```python
from build123d import *

# Parameters (mm, degrees)
EXTRUDE_1_DEPTH = 75
FILLET_1_R      = 3


with BuildPart() as part:
    # Эскиз1 → Вытянуть-Тонкостенный1 (new, symmetric)
    with BuildSketch(Plane.XY):
        Polygon((0, 0), (20, 0), (20, 53), (0, 53), (0, 50), (17, 50), (17, 3), (0, 3), align=None)
    extrude(amount=EXTRUDE_1_DEPTH, both=True)

    # Скругление1
    fillet_1_edges = [part.edges().sort_by_distance(p)[0] for p in [
        (17, 3, 0),
        (17, 50, 0),
    ]]
    fillet(fillet_1_edges, radius=FILLET_1_R)


solid = part.part
```
The model under review builds one solid part; all positions refer to its coordinate system, in mm. A direction names the side the tool comes from. Give positions to 0.01 mm unless a question says otherwise; leave off trailing zeros. Write each loop counter-clockwise with the first axis right and the second up, starting at its lowest first coordinate (ties: lowest second). Pieces come first, ordered by that corner, then holes. Notation, with made-up numbers: (17, 34.25) -> (39, 34.25) arc R22 ccw to (39, 53.25) -> close; hole circle Ø2 at (4.5, 3). An arc over 180 degrees is marked (long way). Answer in a Markdown table with one row per item.
1) Add section C-C on y = 15. State the section outline as (x, z) points.
Worked answers:
| item | result |
|---|---|
| outline | (17, -75) -> (20, -75) -> (20, 75) -> (17, 75) -> close |
2) Add section B-B on z = -44. State the section outline as (x, y) points, plus the area to 3 significant figures.
Worked answers:
| item | result |
|---|---|
| outline | (0, 0) -> (20, 0) -> (20, 53) -> (0, 53) -> (0, 50) -> (14, 50) arc R3 cw to (17, 47) -> (17, 6) arc R3 cw to (14, 3) -> (0, 3) -> close |
| area | 265 mm² |
3) Add section A-A on x = 6.75. State the section outline as (y, z) points.
Worked answers:
| item | result |
|---|---|
| outline | (0, -75) -> (3, -75) -> (3, 75) -> (0, 75) -> close; (50, -75) -> (53, -75) -> (53, 75) -> (50, 75) -> close |
4) Tool access review of faces 5 (the flat face through (7, 3, 1)), 6 (the flat face through (17.4, 28.6, -75)): name each direction out of +Z, -Z, +X, -X, +Y, -Y from which nothing blocks a thin tool from reaching the whole face with its end or side.
Worked answers:
| item | result |
|---|---|
| face 5 | +Z, -Z, -X |
| face 6 | -Z, +X, -X, +Y, -Y |
5) For L1, parallel to Y at x = 9, z = -21; L2, parallel to X at y = 13, z = 67.5; L3, parallel to Y at x = 15, z = -62, list the stretches that pass through material, from the lowest coordinate up. Write a range as [from, to].
Worked answers:
| item | result |
|---|---|
| L1 | [0, 3], [50, 53] |
| L2 | [17, 20] |
| L3 | [0, 3.17], [49.83, 53] |
6) Clearance check with flat-ended pins moving along their axes: P1, Ø2, axis at x = 8, y = 47.5, coming from the -Z side; P2, Ø20.5, axis at y = 36.5, z = 9.5, coming from the -X side. State where each tip first meets the part, or that it passes through.
Worked answers:
| item | result |
|---|---|
| P1 | through |
| P2 | x = 17 |
7) Mouldability with a two-part tool opening along Y and no side actions: class faces 1 (the flat face through (17, 27, 1)), 2 (the flat face through (10, 0, 1)), 3 (the flat face through (20, 26, 1)), 4 (the flat face through (10, 53, 1)) as +Y half, -Y half, draft (parallel to the pull), parting line (faces both ways), or undercut.
Worked answers:
| item | result |
|---|---|
| face 1 | undercut |
| face 2 | -Y half |
| face 3 | draft |
| face 4 | +Y half |
